Read the model definition and answer for the solid it produces. Units are mm, in the model's axes. A direction names the side the tool comes from. Give positions to 0.01 mm unless a question says otherwise; leave off trailing zeros. Loops run counter-clockwise (first coordinate to the right, second up) from the corner with the lowest first, then second, coordinate; pieces in that order, holes last. Notation, with made-up numbers: (44, 50.25) - (56, 50.25) arc R13 ccw to (56, 67.25) - close; hole circle Ø6 at (-33.5, 68). An arc over 180 degrees is marked (long way). Use a Markdown table: item, result. Add a question column.
Item 1: Consider probe 1 along Z at (x, y) = (0, -2.5); probe 2 along X at (y, z) = (-16.75, -24.5); probe 3 along Z at (x, y) = (-32, -16.5). Determine where each line is inside the solid, lowest interval first. Write a range as [from, to].
Item 2: A cutting plane is placed at A-A (z = 0). Determine the outline of the cut face in (x, y).
Item 3: A cutting plane is placed at D-D (x = 32). Determine the outline of the cut face in (y, z).
Item 4: Each of these flat-tipped pins is pushed along its axis until it touches: P1, Ø10, axis at x = -36, y = -3.5, coming from the +Z side; P2, Ø8, axis at y = -17, z = -2, coming from the +X side; P3, Ø3, axis at x = -5, y = -12.5, coming from the -Z side; P4, Ø8, axis at x = 0, z = 55.56, coming from the -Y side. Where does it stop, or does it pass through?
Item 5: A cutting plane is placed at C-C (z = 25). Determine the outline of the cut face in (x, y), plus the area to 3 significant figures.
Item 6: Which of the six approach directions +Z, -Z, +X, -X, +Y, -Y give full straight-line access (tool end or side, diameter ignored) to faces 4 (the face through (33, -25.4, 20)), 5 (the face through (42.397, -15.742, 13.352))?
Item 7: A cutting plane is placed at B-B (x = 0). Determine the outline of the cut face in (y, z), plus the area to 3 significant figures.
Item 8: For a pull along X with two mould halves and no side action, classify faces 1 (the face through (0.656, -3.131, -50.564)), 2 (the face through (-13.77, -3.13, -61.99)), 3 (the face through (-38, -6.35, 24)) as +X half, -X half, draft (parallel to the pull), parting line (faces both ways), or undercut.
from build123d import *

# Parameters (mm, degrees)
F0_R     = 63.5
F0_R_2   = 38.1
F1_DEPTH = 6.35
F2_R     = 44.45
F2_R_2   = 38.1
F3_DEPTH = 19.05
F5_D     = 10.0838


with BuildPart() as f1:
    # F0 (on Front) → F1 (new body)
    with BuildSketch(Plane.XZ):
        Circle(F0_R)
        Circle(F0_R_2, mode=Mode.SUBTRACT)
    extrude(amount=F1_DEPTH)

    # F2 (on face) → F3 (join)
    with BuildSketch(Plane.XZ.offset(6.35)):
        Circle(F2_R)
        Circle(F2_R_2, mode=Mode.SUBTRACT)
    extrude(amount=F3_DEPTH)

    # F5 (through all)
    with Locations(Plane.XZ.offset(6.35)):
        with Locations((0, 55.5625), (55.5625, 0), (-55.5625, 0), (0, -55.5625)):
            Hole(F5_D / 2)


solid = f1.part
Geometry says:
| question | item | result |
|---|---|---|
| 1 | probe 1 | [-63.5, -60.6], [-50.52, -38.1], [38.1, 50.52], [60.6, 63.5] |
| 1 | probe 2 | [-37.09, -29.18], [29.18, 37.09] |
| 1 | probe 3 | [-30.85, -20.68], [20.68, 30.85] |
| 2 | outline | (-63.5, -6.35) - (-60.6, -6.35) - (-60.6, 0) - (-63.5, 0) - close; (-50.52, -6.35) - (-44.45, -6.35) - (-44.45, -25.4) - (-38.1, -25.4) - (-38.1, 0) - (-50.52, 0) - close; (38.1, -25.4) - (44.45, -25.4) - (44.45, -6.35) - (50.52, -6.35) - (50.52, 0) - (38.1, 0) - close; (60.6, -6.35) - (63.5, -6.35) - (63.5, 0) - (60.6, 0) - close |
| 3 | outline | (-25.4, -30.85) - (-6.35, -30.85) - (-6.35, -54.85) - (0, -54.85) - (0, -20.68) - (-25.4, -20.68) - close; (-25.4, 20.68) - (0, 20.68) - (0, 54.85) - (-6.35, 54.85) - (-6.35, 30.85) - (-25.4, 30.85) - close |
| 4 | P1 | z = 55.42 |
| 4 | P2 | x = 44.45 |
| 4 | P3 | z = -44.31 |
| 4 | P4 | through |
| 5 | outline | (-58.37, -6.35) - (-36.75, -6.35) - (-36.75, -25.4) - (-28.75, -25.4) - (-28.75, 0) - (-58.37, 0) - close; (28.75, -25.4) - (36.75, -25.4) - (36.75, -6.35) - (58.37, -6.35) - (58.37, 0) - (28.75, 0) - close |
| 5 | area | 681 mm² |
| 6 | face 4 | +Z, -Z, +X, -X, -Y |
| 6 | face 5 | -Y |
| 7 | outline | (-25.4, -44.45) - (-6.35, -44.45) - (-6.35, -50.52) - (0, -50.52) - (0, -38.1) - (-25.4, -38.1) - close; (-25.4, 38.1) - (0, 38.1) - (0, 50.52) - (-6.35, 50.52) - (-6.35, 44.45) - (-25.4, 44.45) - close; (-6.35, -63.5) - (0, -63.5) - (0, -60.6) - (-6.35, -60.6) - close; (-6.35, 60.6) - (0, 60.6) - (0, 63.5) - (-6.35, 63.5) - close |
| 7 | area | 436 mm² |
| 8 | face 1 | undercut |
| 8 | face 2 | parting line |
| 8 | face 3 | draft |
